from build123d import *

# Parameters (mm, degrees)
SKETCH_W               = 54
SKETCH_H               = 69
SKETCH_R               = 2.1
PAD_DEPTH              = 13
SKETCH001_W            = 4
SKETCH001_H            = 2
POCKET_DEPTH           = 13
LINEARPATTERN_COUNT    = 2
LINEARPATTERN_PITCH    = 25
SKETCH002_R            = 7.7
POCKET001_DEPTH        = 58
SKETCH003_W            = 54
SKETCH003_H            = 15.3
POCKET002_DEPTH        = 6
SKETCH004_W            = 54
SKETCH004_H            = 9
PAD001_DEPTH           = 7
SKETCH005_R            = 0.7
PAD002_DEPTH           = 7
LINEARPATTERN001_COUNT = 13
LINEARPATTERN001_PITCH = 4.166667
SKETCH006_W            = 8
SKETCH006_H            = 10.6
POCKET003_DEPTH        = 7
SKETCH007_W            = 2
SKETCH007_H            = 16
PAD003_DEPTH           = 10
SKETCH008_R            = 6
POCKET004_DEPTH        = 58
SKETCH009_W            = 4
SKETCH009_H            = 22
POCKET005_DEPTH        = 2
CHAMFER_SIZE           = 6
FILLET_R               = 3


with BuildPart() as part:
    # Sketch → Pad (new body)
    with BuildSketch(Plane(origin=(43, 0, 135.5), x_dir=(1, 0, 0), z_dir=(0, 1, 0))):
        with Locations((-46.353792, 17.791164)):
            Rectangle(SKETCH_W, SKETCH_H)
        with Locations((-57.353792, 28.791164)):
            Circle(SKETCH_R, mode=Mode.SUBTRACT)
        with Locations((-35.353792, 28.791164)):
            Circle(SKETCH_R, mode=Mode.SUBTRACT)
        with Locations((-57.353792, 6.791164)):
            Circle(SKETCH_R, mode=Mode.SUBTRACT)
        with Locations((-35.353792, 6.791164)):
            Circle(SKETCH_R, mode=Mode.SUBTRACT)
    extrude(amount=PAD_DEPTH)

    # Sketch001 → Pocket (cut)
    with BuildSketch(Plane(origin=(43, 13, 135.5), x_dir=(1, 0, 0), z_dir=(0, 1, 0))):
        with Locations((-67.353792, 50.291164)):
            Rectangle(SKETCH001_W, SKETCH001_H)
        with Locations((-67.353792, 30.291164)):
            Rectangle(SKETCH001_W, SKETCH001_H)
        with Locations((-67.353792, 5.291164)):
            Rectangle(SKETCH001_W, SKETCH001_H)
        with Locations((-67.353792, -14.708836)):
            Rectangle(SKETCH001_W, SKETCH001_H)
        with Locations((-51.353792, 50.291164)):
            Rectangle(SKETCH001_W, SKETCH001_H)
        with Locations((-51.353792, 30.291164)):
            Rectangle(SKETCH001_W, SKETCH001_H)
        with Locations((-51.353792, 5.291164)):
            Rectangle(SKETCH001_W, SKETCH001_H)
        with Locations((-51.353792, -14.708836)):
            Rectangle(SKETCH001_W, SKETCH001_H)
    pocket = extrude(amount=-POCKET_DEPTH, mode=Mode.SUBTRACT)

    # LinearPattern: Pocket ×2
    with Locations(*[(i * LINEARPATTERN_PITCH, 0, 0) for i in range(1, LINEARPATTERN_COUNT)]):
        add(pocket, mode=Mode.SUBTRACT)

    # Sketch002 → Pocket001 (cut)
    with BuildSketch(Plane(origin=(-30.353792, 0, 135.5), x_dir=(0, 0, 1), z_dir=(-1, 0, 0))):
        with Locations((-40.291164, 11)):
            Circle(SKETCH002_R)
        with Locations((4.708836, 11)):
            Circle(SKETCH002_R)
    extrude(amount=-POCKET001_DEPTH, mode=Mode.SUBTRACT)

    # Sketch003 → Pocket002 (cut)
    with BuildSketch(Plane(origin=(43, 13, 135.5), x_dir=(1, 0, 0), z_dir=(0, 1, 0))):
        with Locations((-46.353792, 17.641164)):
            Rectangle(SKETCH003_W, SKETCH003_H)
    extrude(amount=-POCKET002_DEPTH, mode=Mode.SUBTRACT)

    # Sketch004 → Pad001 (new body)
    with BuildSketch(Plane(origin=(43, 7, 135.5), x_dir=(1, 0, 0), z_dir=(0, 1, 0))):
        with Locations((-46.353792, 19.191164)):
            Rectangle(SKETCH004_W, SKETCH004_H)
    extrude(amount=PAD001_DEPTH)

    # Sketch005 → Pad002 (new body)
    with BuildSketch(Plane(origin=(43, 14, 135.5), x_dir=(1, 0, 0), z_dir=(0, 1, 0))):
        with Locations((-72.353792, 23.691164)):
            Circle(SKETCH005_R)
        with Locations((-70.353792, 23.691164)):
            Circle(SKETCH005_R)
    pad002 = extrude(amount=-PAD002_DEPTH)

    # LinearPattern001: Pad002 ×13
    with Locations(*[(i * LINEARPATTERN001_PITCH, 0, 0) for i in range(1, LINEARPATTERN001_COUNT)]):
        add(pad002)

    # Sketch006 → Pocket003 (cut)
    with BuildSketch(Plane(origin=(43, 14, 135.5), x_dir=(1, 0, 0), z_dir=(0, 1, 0))):
        with Locations((-46.353792, 19.991164)):
            Rectangle(SKETCH006_W, SKETCH006_H)
    extrude(amount=-POCKET003_DEPTH, mode=Mode.SUBTRACT)

    # Sketch007 → Pad003 (new body)
    with BuildSketch(Plane(origin=(43, 13, 135.5), x_dir=(1, 0, 0), z_dir=(0, 1, 0))):
        with Locations((-72.353792, 40.291164)):
            Rectangle(SKETCH007_W, SKETCH007_H)
        with Locations((-46.353792, 40.291164)):
            Rectangle(SKETCH007_W, SKETCH007_H)
        with Locations((-20.353792, 40.291164)):
            Rectangle(SKETCH007_W, SKETCH007_H)
        with Locations((-72.353792, -4.708836)):
            Rectangle(SKETCH007_W, SKETCH007_H)
        with Locations((-46.353792, -4.708836)):
            Rectangle(SKETCH007_W, SKETCH007_H)
        with Locations((-20.353792, -4.708836)):
            Rectangle(SKETCH007_W, SKETCH007_H)
    extrude(amount=-PAD003_DEPTH)

    # Sketch008 → Pocket004 (cut)
    with BuildSketch(Plane(origin=(-30.353792, 0, 135.5), x_dir=(0, 0, 1), z_dir=(-1, 0, 0))):
        with Locations((-40.291164, 11)):
            Circle(SKETCH008_R)
        with Locations((4.708836, 11)):
            Circle(SKETCH008_R)
    extrude(amount=-POCKET004_DEPTH, mode=Mode.SUBTRACT)

    # Sketch009 → Pocket005 (cut)
    with BuildSketch(Plane(origin=(43, 0, 135.5), x_dir=(1, 0, 0), z_dir=(0, -1, 0))):
        with Locations((-67.353792, 4.708836)):
            Rectangle(SKETCH009_W, SKETCH009_H)
        with Locations((-51.353792, 4.708836)):
            Rectangle(SKETCH009_W, SKETCH009_H)
        with Locations((-42.353792, 4.708836)):
            Rectangle(SKETCH009_W, SKETCH009_H)
        with Locations((-26.353792, 4.708836)):
            Rectangle(SKETCH009_W, SKETCH009_H)
        with Locations((-67.353792, -40.291164)):
            Rectangle(SKETCH009_W, SKETCH009_H)
        with Locations((-51.353792, -40.291164)):
            Rectangle(SKETCH009_W, SKETCH009_H)
        with Locations((-42.353792, -40.291164)):
            Rectangle(SKETCH009_W, SKETCH009_H)
        with Locations((-26.353792, -40.291164)):
            Rectangle(SKETCH009_W, SKETCH009_H)
    extrude(amount=-POCKET005_DEPTH, mode=Mode.SUBTRACT)

    # Chamfer
    chamfer_edges = [part.edges().sort_by_distance(p)[0] for p in [
        (23.646208, 10.5, 120.808836),
        (0.646208, 10.5, 120.808836),
        (-7.353792, 10.5, 120.808836),
        (-30.353792, 10.5, 120.808836),
    ]]
    chamfer(chamfer_edges, length=CHAMFER_SIZE)

    # Fillet
    fillet_edges = [part.edges().sort_by_distance(p)[0] for p in [
        (23.646208, 6.5, 83.208836),
        (-30.353792, 6.5, 83.208836),
        (-30.353792, 6.5, 152.208836),
        (23.646208, 6.5, 152.208836),
        (23.646208, 10, 125.508836),
        (-30.353792, 10, 110.208836),
        (-30.353792, 10, 125.508836),
    ]]
    fillet(fillet_edges, radius=FILLET_R)


solid = part.part
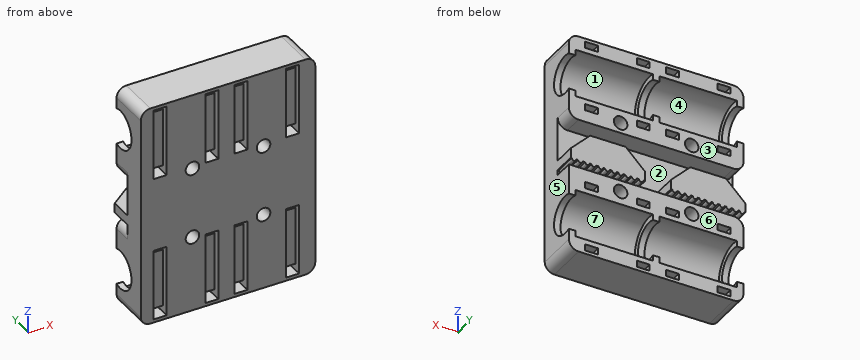
Work out the finished part from the listing and answer in its coordinate system (mm). Face numbers are marked on the shaded views. A direction names the side the tool comes from. Give positions to 0.01 mm unless a question says otherwise; leave off trailing zeros. Order: outer loops, then holes, each group sorted by start corner. A loop starts at its lowest first (then second) coordinate and runs counter-clockwise, first axis right, second up. Notation, with made-up numbers: (-26, 52) -> (-9, 52) arc R27 ccw to (-9, 85) -> close; hole circle Ø3 at (44, 7). An arc over 180 degrees is marked (long way). Answer as a JSON object with one key per item and string values. Group by question number.
1. The mould has two halves that part along X. Classify the marked faces 4, 5, 6 and 7: released by +X, released by -X, zero draft, split by the parting line, or undercut.
2. A tool of negligible diameter and unlimited length cuts with its end or side. For the marked faces 1, 2 and 3, from which of +Z, -Z, +X, -X, +Y, -Y can it reach the whole face along a straight path? Write none if from no direction.
3. Consider line 1 along Z through (x, y) = (-3.5, 11); line 2 along X through (y, z) = (4.75, 144); line 3 along Z through (x, y) = (2, 3). Determine where each line is inside the solid, lowest interval first. Write a range as [from, to].
4. Section C-C on z = 143.5 is taken. Determine the outline of the cut face in (x, y), plus the area to 3 significant figures.
5. Flat-ended cylindrical pins translate along their axes: pin 1 Ø1.5 at (x, z) = (-16.5, 138.5) entering from -Y; pin 2 Ø7 at (x, z) = (-7.5, 85) entering from +Y. Find the tip coordinate at first contact, or state that the pin passes through.
6. Section A-A on y = 11 is taken. Count the separate pieces of the cut face and the enclosed holes in it, plus the area to 3 significant figures.
7. Section B-B on z = 94.5 is taken. Determine the outline of the cut face in (x, y).
Result sheet:
{
 "1": {"face 4": "undercut", "face 5": "released by +X", "face 6": "zero draft", "face 7": "undercut"},
 "2": {"face 1": "none", "face 2": "+Y", "face 3": "+Z, +X, -X, +Y"},
 "3": {"line 1": "z = [83.21, 89.21], [101.21, 110.21], [125.51, 134.21], [146.21, 152.21]", "line 2": "x = [-30.35, -28.35], [-4.35, -2.35], [21.65, 23.65]", "line 3": "z = [83.21, 84.21], [86.21, 104.21], [106.21, 129.21], [131.21, 149.21], [151.21, 152.21]"},
 "4": {"outline": "(-30.35, 0) -> (-26.35, 0) -> (-26.35, 2) -> (-22.35, 2) -> (-22.35, 0) -> (-10.35, 0) -> (-10.35, 2) -> (-6.35, 2) -> (-6.35, 0) -> (-1.35, 0) -> (-1.35, 2) -> (2.65, 2) -> (2.65, 0) -> (14.65, 0) -> (14.65, 2) -> (18.65, 2) -> (18.65, 0) -> (23.65, 0) -> (23.65, 5.98) -> (21.65, 5.98) -> (21.65, 4.04) -> (-2.35, 4.04) -> (-2.35, 5.98) -> (-4.35, 5.98) -> (-4.35, 4.04) -> (-28.35, 4.04) -> (-28.35, 5.98) -> (-30.35, 5.98) -> close", "area": "198 mm^2"},
 "5": {"pin 1": "stops at y = 0", "pin 2": "stops at y = 13"},
 "6": {"separate pieces": "6", "enclosed holes": "20", "area": "1,440 mm^2"},
 "7": {"outline": "(-30.35, 0) -> (-26.35, 0) -> (-26.35, 2) -> (-22.35, 2) -> (-22.35, 0) -> (-10.35, 0) -> (-10.35, 2) -> (-6.35, 2) -> (-6.35, 0) -> (-1.35, 0) -> (-1.35, 2) -> (2.65, 2) -> (2.65, 0) -> (14.65, 0) -> (14.65, 2) -> (18.65, 2) -> (18.65, 0) -> (23.65, 0) -> (23.65, 5.04) -> (21.65, 5.04) -> (21.65, 3.33) -> (-2.35, 3.33) -> (-2.35, 5.04) -> (-4.35, 5.04) -> (-4.35, 3.33) -> (-28.35, 3.33) -> (-28.35, 5.04) -> (-30.35, 5.04) -> close"}
}
